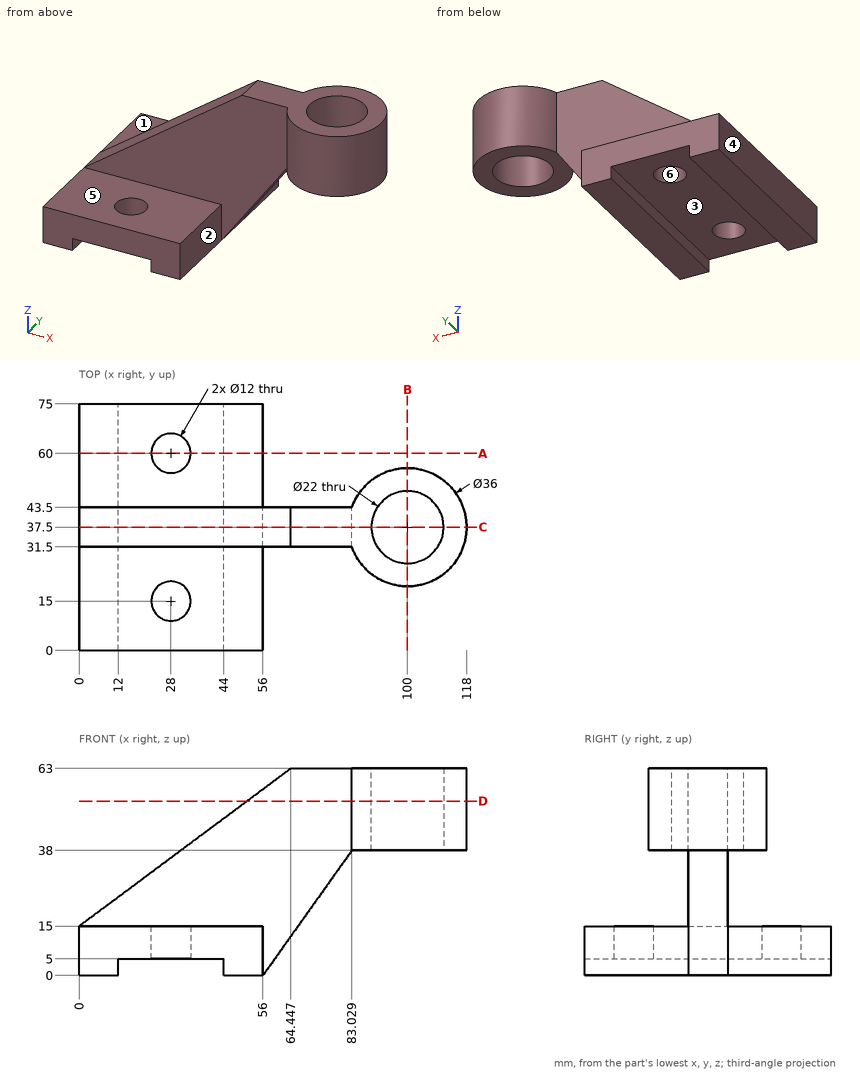
The drawing under review shows one solid part. Ordinate dimensions are in mm from its lowest x, y, z. A direction names the side the tool comes from. Give positions to 0.01 mm unless a question says otherwise; leave off trailing zeros. Loops run counter-clockwise (first coordinate to the right, second up) from the corner with the lowest first, then second, coordinate; pieces in that order, holes last. Notation, with made-up numbers: M 34,-16 L 83,-16 A14 cw 83,6 Z; hole C -28.5,-5.75 d2. An arc over 180 degrees is marked long. Return JSON: item names as keys, results as strings. Group by question number.
Item 1: Insertion check: pin 1 Ø10.5 at (x, y) = (107.5, 46) entering from -Z; pin 2 Ø5 at (y, z) = (53.5, 45) entering from -X (1 decimal); pin 3 Ø10 at (y, z) = (55.5, 10.5) entering from +X. Each pin has a flat end and moves straight along its axis. Give the tip position at first contact, or say it passes through.
Item 2: For probe 1 along Y at (x, z) = (28, 8); probe 2 along Y at (x, z) = (100, 49); probe 3 along Z at (x, y) = (30.5, 25.5), list the stretches that pass through material, from the lowest coordinate up.
Item 3: Mouldability with a two-part tool opening along X and no side actions: class the marked faces 4, 5 and 6 as released by +X, released by -X, zero draft, split by the parting line, or undercut.
Item 4: We need section C-C (y = 37.5). Give the boundary of the cut face in (x, z), and give its area (4 significant figures).
Item 5: We need section B-B (x = 100). Give the boundary of the cut face in (y, z).
Item 6: We need section D-D (z = 53). Give the boundary of the cut face in (x, y).
Item 7: We need section A-A (y = 60). Give the boundary of the cut face in (x, z), and give its area (3 significant figures).
Item 8: Tool access review of the marked faces 1, 2 and 3: name each direction out of +Z, -Z, +X, -X, +Y, -Y from which nothing blocks a thin tool from reaching the whole face with its end or side.
Output:
{
 "1": {"pin 1": "stops at z = 38", "pin 2": "stops at x = 88.1", "pin 3": "stops at x = 56"},
 "2": {"probe 1": "y = 0 to 9, 21 to 54, 66 to 75", "probe 2": "y = 19.5 to 26.5, 48.5 to 55.5", "probe 3": "z = 5 to 15"},
 "3": {"face 4": "released by -X", "face 5": "zero draft", "face 6": "undercut"},
 "4": {"outline": "M 0,0 L 12,0 L 12,5 L 44,5 L 44,0 L 56,0 L 83.03,38 L 89,38 L 89,63 L 64.45,63 L 0,15 Z; M 111,38 L 118,38 L 118,63 L 111,63 Z", "area": "3,335 mm^2"},
 "5": {"outline": "M 19.5,38 L 26.5,38 L 26.5,63 L 19.5,63 Z; M 48.5,38 L 55.5,38 L 55.5,63 L 48.5,63 Z"},
 "6": {"outline": "M 51.02,31.5 L 83.03,31.5 A18 ccw long 83.03,43.5 L 51.02,43.5 Z; hole C 100,37.5 d22"},
 "7": {"outline": "M 0,0 L 12,0 L 12,5 L 22,5 L 22,15 L 0,15 Z; M 34,5 L 44,5 L 44,0 L 56,0 L 56,15 L 34,15 Z", "area": "560 mm^2"},
 "8": {"face 1": "+Z, +X, -X, +Y", "face 2": "+Z, -Z, +X, -Y", "face 3": "-Z, +Y, -Y"}
}
